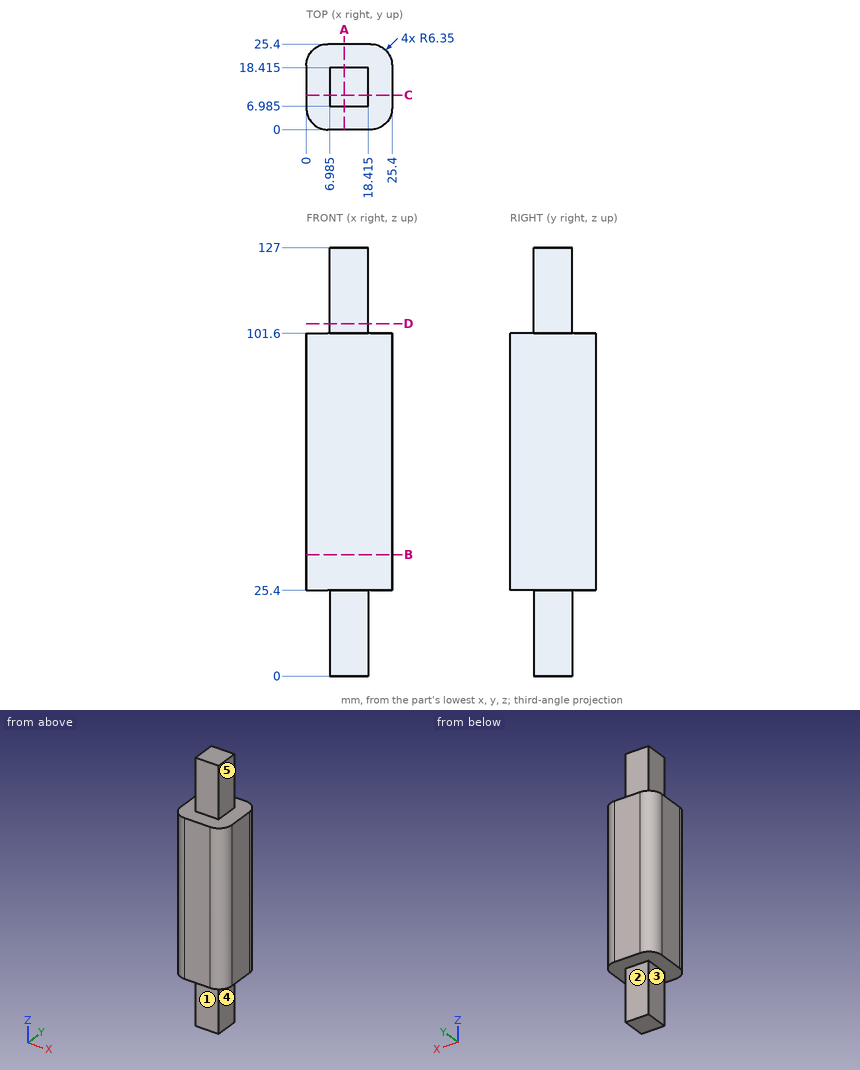
Answer from the drawing. Dimensions are ordinates in mm from the lowest x, y and z of the part. A direction names the side the tool comes from. Round coordinates to 2 decimals unless told otherwise and drop trailing zeros. Write each loop counter-clockwise with the first axis right and the second up, starting at its lowest first coordinate (ties: lowest second). Pieces come first, ordered by that corner, then holes. Notation, with made-up numbers: (80, 72) -> (100, 72) arc R16 cw to (100, 94) -> close; hole circle Ø7 at (77, 41.25). An arc over 180 degrees is marked (long way). Answer in a Markdown table with one row per item. Add a question column.
1) Given P1, Ø3.5, axis at y = 13, z = 7.5, coming from the -X side (3 decimals); P2, Ø2, axis at x = 22, y = 22, coming from the +Z side; P3, Ø1.5, axis at y = 11, z = 34, coming from the -X side; P4, Ø12.5, axis at x = 15, z = 119.5, coming from the +Y side (3 decimals), each flat-ended and moving along its own axis, determine where each tip first touches the part or whether it passes through.
2) Find section D-D, the plane z = 104.5. Determine the outline of the cut face in (x, y) (3 decimals).
3) Find section A-A, the plane x = 11.25. Determine the outline of the cut face in (y, z) (3 decimals), and give its area (3 significant figures).
4) Consider line 1 (Z direction, x = 10.75, y = 5.75); line 2 (X direction, y = 21.5, z = 31.5); line 3 (Y direction, x = 19.25, z = 71.5). Determine where each line is inside the solid, lowest interval first.
5) Find section B-B, the plane z = 36. Determine the outline of the cut face in (x, y), and give its area (3 significant figures).
6) Which of the six approach directions +Z, -Z, +X, -X, +Y, -Y give full straight-line access (tool end or side, diameter ignored) to the marked faces 1, 2, 3, 4 and 5?
Findings below:
| question | item | result |
|---|---|---|
| 1 | P1 | x = 6.985 |
| 1 | P2 | z = 101.6 |
| 1 | P3 | x = 0 |
| 1 | P4 | y = 18.415 |
| 2 | outline | (6.985, 6.985) -> (18.415, 6.985) -> (18.415, 18.415) -> (6.985, 18.415) -> close |
| 3 | outline | (0, 25.4) -> (6.985, 25.4) -> (6.985, 0) -> (18.415, 0) -> (18.415, 25.4) -> (25.4, 25.4) -> (25.4, 101.6) -> (18.415, 101.6) -> (18.415, 127) -> (6.985, 127) -> (6.985, 101.6) -> (0, 101.6) -> close |
| 3 | area | 2,520 mm² |
| 4 | line 1 | 25.4 to 101.6 |
| 4 | line 2 | 0.49 to 24.91 |
| 4 | line 3 | 0 to 25.4 |
| 5 | outline | (0, 6.35) arc R6.35 ccw to (6.35, 0) -> (19.05, 0) arc R6.35 ccw to (25.4, 6.35) -> (25.4, 19.05) arc R6.35 ccw to (19.05, 25.4) -> (6.35, 25.4) arc R6.35 ccw to (0, 19.05) -> close |
| 5 | area | 611 mm² |
| 6 | face 1 | -Z, +X, -X, -Y |
| 6 | face 2 | -Z, +X, -X, +Y |
| 6 | face 3 | -Z, -X, +Y, -Y |
| 6 | face 4 | -Z, +X, +Y, -Y |
| 6 | face 5 | +Z, +X, +Y, -Y |
